Source: three-view drawing plus pictorial views. Frame: mm from the lowest corner of the part. Round coordinates to 2 decimals unless told otherwise and drop trailing zeros. Loops run counter-clockwise (first coordinate to the right, second up) from the corner with the lowest first, then second, coordinate; pieces in that order, holes last. Notation, with made-up numbers: M 12.25,20 L 28.25,20 A10 cw 28.25,38 Z; hole C -16,19 d5. An arc over 180 degrees is marked long. Return JSON: item names as keys, results as strings. Group by question number.
1) Section A-A (y = 56). Output: boundary loops of the cut face in (x, z) (1 decimal).
2) Material intervals for line 1 (Y direction, x = 3, z = 0.65); line 2 (Y direction, x = 16, z = 1.75); line 3 (X direction, y = 39, z = 0.55) (1 decimal), sorted ascending. Write a range as from..to.
3) Section B-B (z = 1.25). Count the separate pieces of the cut face and the enclosed holes in it, plus the area to 3 significant figures.
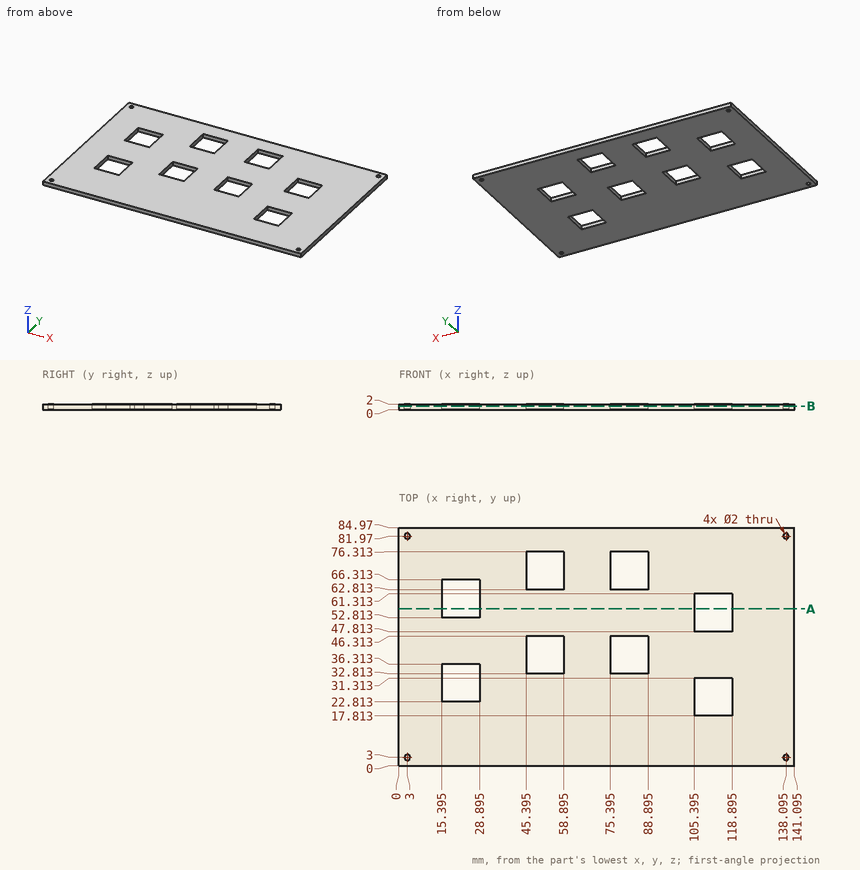
Returned:
{
 "1": {"outline": "M 0,0 L 15.4,0 L 15.4,2 L 0,2 Z; M 28.9,0 L 105.4,0 L 105.4,2 L 28.9,2 Z; M 118.9,0 L 141.1,0 L 141.1,2 L 118.9,2 Z"},
 "2": {"line 1": "y = 0..2, 4..80.97, 82.97..84.97", "line 2": "y = 0..22.81, 36.31..52.81, 66.31..84.97", "line 3": "x = 0..45.4, 58.9..75.4, 88.9..141.1"},
 "3": {"separate pieces": "1", "enclosed holes": "12", "area": "10,500 mm^2"}
}
